from build123d import *

# Parameters (mm, degrees)
BOSS_EXTRUDE1_DEPTH = 2.38125
FILLET1_R           = 3.175
CUT_EXTRUDE1_DEPTH  = 69.433035528


with BuildPart() as part:
    # Sketch1 → Boss-Extrude1 (new body)
    with BuildSketch(Plane.XY):
        Polygon((0, 0), (11.43, 0), (11.43, 13.97), (52.07, 13.97), (52.07, 0), (63.5, 0), (63.5, 25.4), (0, 25.4), align=None)
    extrude(amount=BOSS_EXTRUDE1_DEPTH)

    # Fillet1
    fillet1_edges = [part.edges().sort_by_distance(p)[0] for p in [
        (52.07, 13.97, 1.190625),
        (11.43, 13.97, 1.190625),
    ]]
    fillet(fillet1_edges, radius=FILLET1_R)

    # Sketch2 → Cut-Extrude1 (cut, through all)
    with BuildSketch(Plane.XY.offset(2.38125)):
        Polygon((0, 25.4), (0, 21.471137947), (3.928862053, 25.4), align=None)
        Polygon((63.5, 25.4), (59.571137947, 25.4), (63.5, 21.471137947), align=None)
    extrude(amount=-CUT_EXTRUDE1_DEPTH, mode=Mode.SUBTRACT)


solid = part.part
CAD build for the part. Positions are in the model's coordinates, mm. A direction names the side the tool comes from. Coordinates: 2 decimals unless noted, no trailing zeros. Write each loop counter-clockwise with the first axis right and the second up, starting at its lowest first coordinate (ties: lowest second). Pieces come first, ordered by that corner, then holes. Notation, with made-up numbers: M 12,-25.75 L 60,-25.75 A28 ccw 60,-0.75 Z; hole C 44,23.5 d2. An arc over 180 degrees is marked long. Answer as a JSON object with one key per item and string values. Group by question number.
1) Tool access for faces 5 (the face through (12.34, 13.02, 1.21)), 6 (the face through (31, 16, 2.381)): list every direction of +Z, -Z, +X, -X, +Y, -Y with a clear straight run to the whole face (end or side of a thin tool).
2) Mould opens along X. For faces 1 (the face through (0, 11, 1)), 2 (the face through (11.43, 5, 1)), 3 (the face through (51.12, 13.06, 1.21)), 4 (the face through (31, 16, 0)) say: +X half, -X half, draft (parallel to the pull), parting line (faces both ways), or undercut.
3) Wall check: line 1 (X direction, y = 2.75, z = 0.35); line 2 (Y direction, x = 16.5, z = 0.9); line 3 (X direction, y = 12, z = 1.55). Give the ranges that are in metal, low to high. Write a range as from..to.
4) Pin check, flat tips, straight feed: pin 1 Ø1 at (x, z) = (25, 2) entering from -Y; pin 2 Ø5 at (x, y) = (49.5, 11.5) entering from +Z. Stop position of each tip, or through.
5) Saw through at B-B (z = 0.9). Write the cut outline in (x, y) (3 decimals).
6) Saw through at A-A (y = 8). Write the cut outline in (x, z), plus the area to 3 significant figures.
7) Saw through at C-C (x = 39.5). Write the cut outline in (y, z).
Values follow:
{
 "1": {"face 5": "+Z, -Z, -Y", "face 6": "+Z, +X, -X, +Y, -Y"},
 "2": {"face 1": "-X half", "face 2": "undercut", "face 3": "undercut", "face 4": "draft"},
 "3": {"line 1": "x = 0..11.43, 52.07..63.5", "line 2": "y = 13.97..25.4", "line 3": "x = 0..11.67, 51.83..63.5"},
 "4": {"pin 1": "stops at y = 13.97", "pin 2": "stops at z = 2.38"},
 "5": {"outline": "M 0,0 L 11.43,0 L 11.43,10.795 A3.175 cw 14.605,13.97 L 48.895,13.97 A3.175 cw 52.07,10.795 L 52.07,0 L 63.5,0 L 63.5,21.471 L 59.571,25.4 L 3.929,25.4 L 0,21.471 Z"},
 "6": {"outline": "M 0,0 L 11.43,0 L 11.43,2.38 L 0,2.38 Z; M 52.07,0 L 63.5,0 L 63.5,2.38 L 52.07,2.38 Z", "area": "54.4 mm2"},
 "7": {"outline": "M 13.97,0 L 25.4,0 L 25.4,2.38 L 13.97,2.38 Z"}
}
